For this review, take the finished solid that the model builds, in its own axes (mm). A direction names the side the tool comes from. Give positions to 0.01 mm unless a question says otherwise; leave off trailing zeros. Loops run counter-clockwise (first coordinate to the right, second up) from the corner with the lowest first, then second, coordinate; pieces in that order, holes last.
```python
from build123d import *
from build123d import SkipClean  # not in build123d's __all__

# Parameters (mm, degrees)
F0_R           = 1.0795
F1_DEPTH       = 2
F3_DEPTH       = 19.9898
F4_R           = 0.508
F5_R           = 0.6
F6_DEPTH       = 28.0045
F7_R           = 1.7
F7_R_2         = 0.6
F8_DEPTH       = 1.016
F9_R           = 1.7
F9_R_2         = 0.6
F10_DEPTH      = 1.016
F12_DEPTH      = 15.01875
F12_DEPTH_BACK = 15.01875


# Not quite as in the source:
# - after a boolean that leaves OpenCascade's solid faulty, fix() repairs it


with BuildPart() as f1:
    # F0 (on Front) → F1 (new body)
    with BuildSketch(Plane.XZ):
        with BuildLine():
            Line((8.92175, 11.43), (-8.92175, 11.43))
            ThreePointArc((-8.92175, 11.43), (-12.5138524484, 9.9421024484), (-14.00175, 6.35))
            Line((-14.00175, 6.35), (-14.00175, -6.35))
            ThreePointArc((-14.00175, -6.35), (-12.5138524484, -9.9421024484), (-8.92175, -11.43))
            Line((-8.92175, -11.43), (8.92175, -11.43))
            ThreePointArc((8.92175, -11.43), (12.5138524484, -9.9421024484), (14.00175, -6.35))
            Line((14.00175, -6.35), (14.00175, 6.35))
            ThreePointArc((14.00175, 6.35), (12.5138524484, 9.9421024484), (8.92175, 11.43))
        make_face()
        with Locations((-9.9949, 0)):
            Circle(F0_R, mode=Mode.SUBTRACT)
        with BuildLine():
            ThreePointArc((-7.62, 5.9055), (-7.0248409794, 7.3423409794), (-5.588, 7.9375))
            Line((-5.588, 7.9375), (5.588, 7.9375))
            ThreePointArc((5.588, 7.9375), (7.0248409794, 7.3423409794), (7.62, 5.9055))
            Line((7.62, 5.9055), (7.62, -5.9055))
            ThreePointArc((7.62, -5.9055), (7.0248409794, -7.3423409794), (5.588, -7.9375))
            Line((5.588, -7.9375), (-5.588, -7.9375))
            ThreePointArc((-5.588, -7.9375), (-7.0248409794, -7.3423409794), (-7.62, -5.9055))
            Line((-7.62, -5.9055), (-7.62, 5.9055))
        make_face(mode=Mode.SUBTRACT)
        with Locations((9.9949, 0)):
            Circle(F0_R, mode=Mode.SUBTRACT)
    extrude(amount=F1_DEPTH)

    # F2 (on face) → F3 (join)
    with BuildSketch(Plane.XZ.offset(2)):
        with BuildLine():
            Line((8.92175, 11.43), (-8.92175, 11.43))
            ThreePointArc((-8.92175, 11.43), (-12.5138524484, 9.9421024484), (-14.00175, 6.35))
            Line((-14.00175, 6.35), (-14.00175, -6.35))
            ThreePointArc((-14.00175, -6.35), (-12.5138524484, -9.9421024484), (-8.92175, -11.43))
            Line((-8.92175, -11.43), (8.92175, -11.43))
            ThreePointArc((8.92175, -11.43), (12.5138524484, -9.9421024484), (14.00175, -6.35))
            Line((14.00175, -6.35), (14.00175, 6.35))
            ThreePointArc((14.00175, 6.35), (12.5138524484, 9.9421024484), (8.92175, 11.43))
        make_face()
        with BuildLine():
            ThreePointArc((-12.98575, 4.064), (-11.1258780605, 8.5541280605), (-6.63575, 10.414))
            Line((-6.63575, 10.414), (6.63575, 10.414))
            ThreePointArc((6.63575, 10.414), (11.1258780605, 8.5541280605), (12.98575, 4.064))
            Line((12.98575, 4.064), (12.98575, -4.064))
            ThreePointArc((12.98575, -4.064), (11.1258780605, -8.5541280605), (6.63575, -10.414))
            Line((6.63575, -10.414), (-6.63575, -10.414))
            ThreePointArc((-6.63575, -10.414), (-11.1258780605, -8.5541280605), (-12.98575, -4.064))
            Line((-12.98575, -4.064), (-12.98575, 4.064))
        make_face(mode=Mode.SUBTRACT)
    extrude(amount=F3_DEPTH)

    # F4
    f4_edges = [f1.edges().sort_by_distance(p)[0] for p in [
        (-11.125878, -2, -8.554128),
        (-12.98575, -2, 0),
        (-11.125878, -2, 8.554128),
        (0, -2, 10.414),
        (11.125878, -2, 8.554128),
        (12.98575, -2, 0),
        (11.125878, -2, -8.554128),
        (0, -2, -10.414),
        (-11.0744, -2, 0),
        (-7.62, -2, 0),
        (-7.024841, -2, -7.342341),
        (-7.024841, -2, 7.342341),
        (0, -2, -7.9375),
        (0, -2, 7.9375),
        (7.024841, -2, -7.342341),
        (7.024841, -2, 7.342341),
        (7.62, -2, 0),
        (8.9154, -2, 0),
    ]]
    fillet(f4_edges, radius=F4_R)

    # F5 (on face) → F6 (cut, through all)
    with BuildSketch(Plane.YZ.offset(14.00175)):
        with Locations((-8, 0)):
            Circle(F5_R)
        with Locations((-16, 0)):
            Circle(F5_R)
    extrude(amount=-F6_DEPTH, mode=Mode.SUBTRACT)

    # F7 (on face) → F8 (join)
    with BuildSketch(Plane.YZ.offset(14.00175)):
        with Locations((-8, 0)):
            Circle(F7_R)
        with Locations((-8, 0)):
            Circle(F7_R_2, mode=Mode.SUBTRACT)
        with Locations((-16, 0)):
            Circle(F7_R)
        with Locations((-16, 0)):
            Circle(F7_R_2, mode=Mode.SUBTRACT)
    extrude(amount=F8_DEPTH)

    # F9 (on face) → F10 (join)
    with BuildSketch(Plane(origin=(-14.00175, 0, 0), x_dir=(0, -1, 0), z_dir=(-1, 0, 0))):
        with Locations((16, 0)):
            Circle(F9_R)
        with Locations((16, 0)):
            Circle(F9_R_2, mode=Mode.SUBTRACT)
        with Locations((8, 0)):
            Circle(F9_R)
        with Locations((8, 0)):
            Circle(F9_R_2, mode=Mode.SUBTRACT)
    with SkipClean():  # cleaning this boolean's faces spoils the solid; the shape is the same uncleaned
        extrude(amount=F10_DEPTH)

    # F11 (on Right) → F12 (cut, two sides)
    with BuildSketch(Plane.YZ) as f12_sk:
        with BuildLine():
            ThreePointArc((-20.9493351826, -2.8575), (-21.715, 0), (-20.9493351826, 2.8575))
            Line((-20.9493351826, 2.8575), (-14.935231149, 13.2742337482))
            Line((-14.935231149, 13.2742337482), (-27.6412566526, 12.4483415457))
            Line((-27.6412566526, 12.4483415457), (-27.6412566526, -22.2988429875))
            Line((-27.6412566526, -22.2988429875), (-9.7248705754, -22.2988429875))
            Line((-9.7248705754, -22.2988429875), (-20.9493351826, -2.8575))
        make_face()
    extrude(amount=-F12_DEPTH, mode=Mode.SUBTRACT)
    extrude(f12_sk.sketch, amount=F12_DEPTH_BACK, mode=Mode.SUBTRACT)

    add(f1.part.fix(), mode=Mode.REPLACE)


solid = f1.part
```
Q1. Machinability: for faces 1 (the cylindrical face through (-7.009, -0.736, -7.358)), 2 (the cylindrical face through (11.175, -9.285, -8.504)), 3 (the cylindrical face through (12.553, -9.334, 9.902)), 4 (the cylindrical face through (14.5, -9.35, -1.03)), 5 (the cylindrical face through (-14.5, -17.57, -0.65)), which of the approach directions +Z, -Z, +X, -X, +Y, -Y give a long, thin tool a straight path to every point of the face, cutting with its end or side? Answer none if there is none.
Answers:
face 1: +Y, -Y
face 2: -Y
face 3: +Z, +X, +Y, -Y
face 4: +X
face 5: -X
Q2. For pin 1 Ø2 at (y, z) = (-8.5, -8.5) entering from +X; pin 2 Ø10 at (x, z) = (3, 3) entering from -Y; pin 3 Ø12 at (x, z) = (4, 6) entering from -Y, all flat-tipped, find the tip position at first contact; note any pin that passes through.
Answers:
pin 1: stops at x = 13.87
pin 2: stops at y = -1.98
pin 3: stops at y = -16.71
Q3. For probe 1 along Y at (x, z) = (-13.3, 0) (3 decimals); probe 2 along X at (y, z) = (-9, -3); probe 3 along Z at (x, y) = (1, -3.25), list the stretches that pass through material, from the lowest coordinate up.
Answers:
probe 1: y = -21.715 to -16.6, -15.4 to -8.6, -7.4 to 0
probe 2: x = -14 to -12.99, 12.99 to 14
probe 3: z = -11.43 to -10.41, 10.41 to 11.43
Q4. Consider section C-C on z = 3.5. Give the boundary of the cut face in (x, y), plus the area to 3 significant figures.
Answers:
outline: (-14, -20.58) - (-12.99, -20.58) - (-12.99, -2.51) arc R0.51 cw to (-12.48, -2) - (-8.13, -2) arc R0.51 ccw to (-7.62, -1.49) - (-7.62, 0) - (-14, 0) - close; (7.62, -1.49) arc R0.51 ccw to (8.13, -2) - (12.48, -2) arc R0.51 cw to (12.99, -2.51) - (12.99, -20.58) - (14, -20.58) - (14, 0) - (7.62, 0) - close
area: 63.3 mm2
Q5. Consider section D-D on y = -4.5. Give the boundary of the cut face in (x, z), plus the area to 3 significant figures.
Answers:
outline: (-14, -6.35) arc R5.08 ccw to (-8.92, -11.43) - (8.92, -11.43) arc R5.08 ccw to (14, -6.35) - (14, 6.35) arc R5.08 ccw to (8.92, 11.43) - (-8.92, 11.43) arc R5.08 ccw to (-14, 6.35) - close; hole (-12.99, -4.06) arc R6.35 ccw to (-6.64, -10.41) - (6.64, -10.41) arc R6.35 ccw to (12.99, -4.06) - (12.99, 4.06) arc R6.35 ccw to (6.64, 10.41) - (-6.64, 10.41) arc R6.35 ccw to (-12.99, 4.06) - close
area: 112 mm2
Q6. Consider section B-B on x = -2. Give the boundary of the cut face in (y, z), plus the area to 3 significant figures.
Answers:
outline: (-16.59, -10.41) - (-16, -11.43) - (0, -11.43) - (0, -7.94) - (-1.49, -7.94) arc R0.51 ccw to (-2, -8.45) - (-2, -9.91) arc R0.51 cw to (-2.51, -10.41) - close; (-16.59, 10.41) - (-2.51, 10.41) arc R0.51 cw to (-2, 9.91) - (-2, 8.45) arc R0.51 ccw to (-1.49, 7.94) - (0, 7.94) - (0, 11.43) - (-16, 11.43) - close
area: 43.0 mm2
Q7. Mouldability with a two-part tool opening along Y and no side actions: class faces 6 (the flat face through (-12.986, -12, 0)), 7 (the cylindrical face through (14.5, -14.43, -0.65)) as +Y half, -Y half, draft (parallel to the pull), parting line (faces both ways), or undercut.
Answers:
face 6: draft
face 7: undercut
